Could you check a few things on this model? Use its own coordinates, in mm. Face numbers are marked on the shaded views. Coordinates: 2 decimals unless noted, no trailing zeros. Write each loop counter-clockwise with the first axis right and the second up, starting at its lowest first coordinate (ties: lowest second). Pieces come first, ordered by that corner, then holes.
```python
from build123d import *

# Parameters (mm, degrees)
SKETCH2_W             = 5
SKETCH2_H             = 10
BOSS_EXTRUDE1_DEPTH   = 27
SKETCH2_W_2           = 10
SKETCH2_H_2           = 5
BOSS_EXTRUDE1_2_DEPTH = 27
BOSS_EXTRUDE1_3_DEPTH = 27
BOSS_EXTRUDE1_4_DEPTH = 27
SKETCH3_W             = 165
SKETCH3_H             = 55.28
BOSS_EXTRUDE2_DEPTH   = 3
SKETCH4_W             = 10
SKETCH4_H             = 3.86
BOSS_EXTRUDE3_DEPTH   = 3
SKETCH5_W             = 10
SKETCH5_H             = 5
BOSS_EXTRUDE4_DEPTH   = 10
SKETCH7_W             = 5
SKETCH7_H             = 10
BOSS_EXTRUDE5_DEPTH   = 10
SKETCH8_R             = 1.73
CUT_EXTRUDE1_DEPTH    = 6


with BuildPart() as part:
    # Sketch2 → Boss-Extrude1 (new body)
    with BuildSketch(Plane.XY):
        with Locations((-74.585, 0)):
            Rectangle(SKETCH2_W, SKETCH2_H)
    extrude(amount=BOSS_EXTRUDE1_DEPTH)



with BuildPart() as body_2:
    # Sketch2 → Boss-Extrude1 2 (new body)
    with BuildSketch(Plane.XY):
        with Locations((0, 29)):
            Rectangle(SKETCH2_W_2, SKETCH2_H_2)
    extrude(amount=BOSS_EXTRUDE1_2_DEPTH)


with BuildPart() as body_3:
    # Sketch2 → Boss-Extrude1 3 (new body)
    with BuildSketch(Plane.XY):
        with Locations((74.585, 0)):
            Rectangle(SKETCH2_W, SKETCH2_H)
    extrude(amount=BOSS_EXTRUDE1_3_DEPTH)


with BuildPart() as body_4:
    # Sketch2 → Boss-Extrude1 4 (new body)
    with BuildSketch(Plane.XY):
        with Locations((0, -29)):
            Rectangle(SKETCH2_W_2, SKETCH2_H_2)
    extrude(amount=BOSS_EXTRUDE1_4_DEPTH)


with BuildPart() as part_1:
    add(part.part)

    add(body_2.part)  # Boss-Extrude2 merges body 2

    add(body_3.part)  # Boss-Extrude2 merges body 3

    add(body_4.part)  # Boss-Extrude2 merges body 4
    # Sketch3 → Boss-Extrude2 (add)
    with BuildSketch(Plane.XY.offset(27)):
        Rectangle(SKETCH3_W, SKETCH3_H)
    extrude(amount=BOSS_EXTRUDE2_DEPTH)

    # Sketch4 → Boss-Extrude3 (add)
    with BuildSketch(Plane.XY.offset(27)):
        with Locations((0, 29.57)):
            Rectangle(SKETCH4_W, SKETCH4_H)
        with Locations((0, -29.57)):
            Rectangle(SKETCH4_W, SKETCH4_H)
    extrude(amount=BOSS_EXTRUDE3_DEPTH)

    # Sketch5 → Boss-Extrude4 (add)
    with BuildSketch(Plane(origin=(0, 5, 0), x_dir=(1, 0, 0), z_dir=(0, 1, 0))):
        with Locations((-82.085, -2.5)):
            Rectangle(SKETCH5_W, SKETCH5_H)
        with Locations((82.085, -2.5)):
            Rectangle(SKETCH5_W, SKETCH5_H)
    extrude(amount=-BOSS_EXTRUDE4_DEPTH)

    # Sketch7 → Boss-Extrude5 (add)
    with BuildSketch(Plane.ZY.offset(5)):
        with Locations((2.5, 36.5)):
            Rectangle(SKETCH7_W, SKETCH7_H)
        with Locations((2.5, -36.5)):
            Rectangle(SKETCH7_W, SKETCH7_H)
    extrude(amount=-BOSS_EXTRUDE5_DEPTH)

    # Sketch8 → Cut-Extrude1 (cut, through all)
    with BuildSketch(Plane.XY.offset(5)):
        with Locations((-82.085, 0)):
            Circle(SKETCH8_R)
        with Locations((0, -36.5)):
            Circle(SKETCH8_R)
        with Locations((82.085, 0)):
            Circle(SKETCH8_R)
        with Locations((0, 36.5)):
            Circle(SKETCH8_R)
    extrude(amount=-CUT_EXTRUDE1_DEPTH, mode=Mode.SUBTRACT)


solid = part_1.part
```
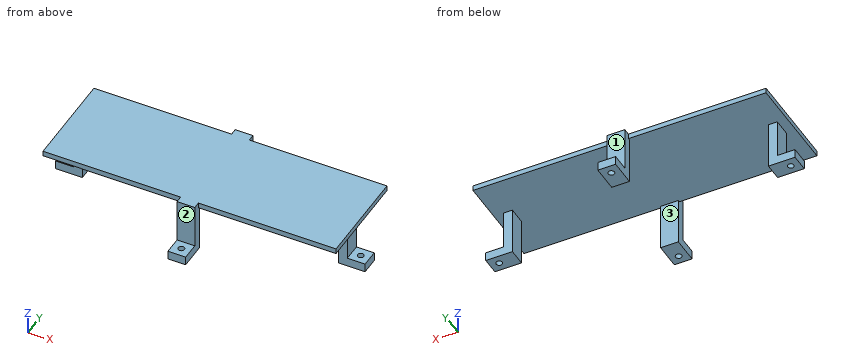
1. Please list where these lines run through material, in increasing order: line 1 along Y through (x, z) = (0, 1.2); line 2 along Z through (x, y) = (6, -22); line 3 along Y through (x, z) = (-78, 3).
Verdict:
line 1: y = -41.5 to -38.23, -34.77 to -26.5, 26.5 to 34.77, 38.23 to 41.5
line 2: z = 27 to 30
line 3: y = -5 to 5
2. If we mould it in two halves opening along Y, with no side actions, what happens to the marked faces 1, 2 and 3? For each: pulls with the +Y half, pulls with the -Y half, needs draft (parallel to the pull), parting line crosses it, or undercut.
Verdict:
face 1: pulls with the +Y half
face 2: pulls with the -Y half
face 3: undercut
3. I want a section at D-D on y = 36.5. Please give me the cut outline in (x, z).
Verdict:
outline: (-5, 0) - (-1.73, 0) - (-1.73, 5) - (-5, 5) - close; (1.73, 0) - (5, 0) - (5, 5) - (1.73, 5) - close
4. For pin 1 (5 mm diameter, centred on x = 2, z = 20, fed in from -Y); pin 2 (5 mm diameter, centred on y = -1.5, z = 17.5, fed in from +X) (3 decimals); pin 3 (4.5 mm diameter, centred on x = 0, y = 36.5, fed in from +Z), each with a flat end and sliding along its axis, tell me the tip position at first contact or that it passes through.
Verdict:
pin 1: stops at y = -31.5
pin 2: stops at x = 77.085
pin 3: stops at z = 5
5. I want a section at A-A on y = 0. Please give me the cut outline in (x, z) (3 decimals), plus the area to 3 significant figures.
Verdict:
outline: (-87.085, 0) - (-83.815, 0) - (-83.815, 5) - (-87.085, 5) - close; (-82.5, 27) - (-77.085, 27) - (-77.085, 5) - (-80.355, 5) - (-80.355, 0) - (-72.085, 0) - (-72.085, 27) - (72.085, 27) - (72.085, 0) - (80.355, 0) - (80.355, 5) - (77.085, 5) - (77.085, 27) - (82.5, 27) - (82.5, 30) - (-82.5, 30) - close; (83.815, 0) - (87.085, 0) - (87.085, 5) - (83.815, 5) - close
area: 830 mm2
6. I want a section at C-C on x = 0. Please give me the cut outline in (y, z), plus the area to 3 significant figures.
Verdict:
outline: (-41.5, 0) - (-38.23, 0) - (-38.23, 5) - (-41.5, 5) - close; (-34.77, 0) - (-26.5, 0) - (-26.5, 27) - (26.5, 27) - (26.5, 0) - (34.77, 0) - (34.77, 5) - (31.5, 5) - (31.5, 30) - (-31.5, 30) - (-31.5, 5) - (-34.77, 5) - close; (38.23, 0) - (41.5, 0) - (41.5, 5) - (38.23, 5) - close
area: 524 mm2
7. I want a section at B-B on z = 19.75. Please give me the cut outline in (x, y) (3 decimals), plus the area to 3 significant figures.
Verdict:
outline: (-77.085, -5) - (-72.085, -5) - (-72.085, 5) - (-77.085, 5) - close; (-5, -31.5) - (5, -31.5) - (5, -26.5) - (-5, -26.5) - close; (-5, 26.5) - (5, 26.5) - (5, 31.5) - (-5, 31.5) - close; (72.085, -5) - (77.085, -5) - (77.085, 5) - (72.085, 5) - close
area: 200 mm2
